```python
from build123d import *

# Parameters (mm, degrees)
SKETCH1_W           = 12
SKETCH1_H           = 10
BOSS_EXTRUDE1_DEPTH = 14.6
SKETCH2_W           = 1
SKETCH2_H           = 5.5
BOSS_EXTRUDE2_DEPTH = 0.5
SKETCH4_R           = 1.5
BOSS_EXTRUDE3_DEPTH = 5.5
SKETCH5_R           = 2.05
BOSS_EXTRUDE4_DEPTH = 0.5
CUT_EXTRUDE1_DEPTH  = 0.5
SKETCH7_R           = 2.5
CUT_EXTRUDE2_DEPTH  = 11
SKETCH9_R           = 3
SKETCH9_R_2         = 2.5
BOSS_EXTRUDE5_DEPTH = 1.6


with BuildPart() as part:
    # Sketch1 → Boss-Extrude1 (new body)
    with BuildSketch(Plane.XY):
        Rectangle(SKETCH1_W, SKETCH1_H)
    extrude(amount=BOSS_EXTRUDE1_DEPTH)

    # Sketch2 → Boss-Extrude2 (add)
    with BuildSketch(Plane.XY.offset(14.6)):
        with Locations((-5.5, 0)):
            Rectangle(SKETCH2_W, SKETCH2_H)
        with Locations((5.5, 0)):
            Rectangle(SKETCH2_W, SKETCH2_H)
    extrude(amount=BOSS_EXTRUDE2_DEPTH)

    # Sketch4 → Boss-Extrude3 (add)
    with BuildSketch(Plane(origin=(0, 0, 0), x_dir=(-1, 0, 0), z_dir=(0, 0, -1))):
        Circle(SKETCH4_R)
    extrude(amount=BOSS_EXTRUDE3_DEPTH)

    # Sketch5 → Boss-Extrude4 (add)
    with BuildSketch(Plane(origin=(0, 0, 0), x_dir=(-1, 0, 0), z_dir=(0, 0, -1))):
        Circle(SKETCH5_R)
    extrude(amount=BOSS_EXTRUDE4_DEPTH)

    # Sketch6 → Cut-Extrude1 (cut)
    with BuildSketch(Plane(origin=(0, 0, 0), x_dir=(-1, 0, 0), z_dir=(0, 0, -1))):
        with BuildLine():
            Line((-5.022000054, 4.19344844), (-4.356935952, 4.19344844))
            Line((-4.356935952, 4.19344844), (-3.752769285, 2.614121517))
            Line((-3.752769285, 2.614121517), (-3.198682747, 4.19344844))
            Line((-3.198682747, 4.19344844), (-2.534820567, 4.19344844))
            Line((-2.534820567, 4.19344844), (-2.534820567, 4.090884337))
            Line((-2.534820567, 4.090884337), (-2.697080183, 4.090884337))
            add(Edge.make_bspline(
                [(-2.697080183, 4.090884337), (-2.710316809, 4.090636556), (-2.734492679, 4.090183998), (-2.76728752, 4.085652982), (-2.793244282, 4.077989549), (-2.813274161, 4.066597021), (-2.826894921, 4.049870677), (-2.8359508, 4.029264042), (-2.841554988, 4.004099098), (-2.842176045, 3.985816116), (-2.842512875, 3.975900363)],
                knots=[0, 0, 0, 0, 1.461409083, 2.669172297, 3.644102285, 4.438396511, 5.171145089, 5.982913306, 6.9060355, 8, 8, 8, 8], degree=3))
            Line((-2.842512875, 3.975900363), (-2.842512875, 2.394570235))
            add(Edge.make_bspline(
                [(-2.842512875, 2.394570235), (-2.842050819, 2.387038144), (-2.841173668, 2.372739479), (-2.834447891, 2.352433769), (-2.823099881, 2.334952111), (-2.806557353, 2.320282642), (-2.784561689, 2.309069969), (-2.756555778, 2.301303429), (-2.722335078, 2.296750977), (-2.697362885, 2.296271709), (-2.683859029, 2.296012542)],
                knots=[0, 0, 0, 0, 0.852734016, 1.618801414, 2.395714484, 3.189123744, 4.096684287, 5.169862416, 6.469586829, 8, 8, 8, 8], degree=3))
            Line((-2.683859029, 2.296012542), (-2.534820567, 2.296012542))
            Line((-2.534820567, 2.296012542), (-2.534820567, 2.19344844))
            Line((-2.534820567, 2.19344844), (-3.432256465, 2.19344844))
            Line((-3.432256465, 2.19344844), (-3.432256465, 2.296012542))
            Line((-3.432256465, 2.296012542), (-3.265189157, 2.296012542))
            add(Edge.make_bspline(
                [(-3.265189157, 2.296012542), (-3.253950106, 2.296245463), (-3.232932895, 2.296681029), (-3.203686174, 2.301738527), (-3.179094381, 2.310536297), (-3.158974617, 2.322618715), (-3.143443119, 2.337663858), (-3.132382481, 2.354803918), (-3.125466503, 2.374031717), (-3.124871883, 2.387565999), (-3.124564157, 2.394570235)],
                knots=[0, 0, 0, 0, 1.394235928, 2.607244209, 3.666761408, 4.619311681, 5.498637875, 6.326439516, 7.133902247, 8, 8, 8, 8], degree=3))
            Line((-3.124564157, 2.394570235), (-3.124564157, 4.09208626))
            Line((-3.124564157, 4.09208626), (-3.791230824, 2.19344844))
            Line((-3.791230824, 2.19344844), (-3.888987234, 2.19344844))
            Line((-3.888987234, 2.19344844), (-4.611743644, 4.08407344))
            Line((-4.611743644, 4.08407344), (-4.611743644, 2.631349081))
            add(Edge.make_bspline(
                [(-4.611743644, 2.631349081), (-4.611377469, 2.611036444), (-4.610694083, 2.573127352), (-4.605325483, 2.520247499), (-4.596108802, 2.475353065), (-4.582524113, 2.437834201), (-4.564432022, 2.407070341), (-4.544422056, 2.379994045), (-4.520414227, 2.357133819), (-4.492696269, 2.33684315), (-4.45794728, 2.320895889), (-4.41471004, 2.309573563), (-4.362603697, 2.300270875), (-4.324529352, 2.297501845), (-4.304051336, 2.296012542)],
                knots=[0, 0, 0, 0, 1.387005521, 2.588542367, 3.624266538, 4.510231893, 5.298685798, 6.05383917, 6.802021236, 7.553697037, 8.390065714, 9.394768359, 10.598794723, 12, 12, 12, 12], degree=3))
            Line((-4.304051336, 2.296012542), (-4.304051336, 2.19344844))
            Line((-4.304051336, 2.19344844), (-5.022000054, 2.19344844))
            Line((-5.022000054, 2.19344844), (-5.022000054, 2.296012542))
            add(Edge.make_bspline(
                [(-5.022000054, 2.296012542), (-5.007558595, 2.297187721), (-4.97993619, 2.299435504), (-4.940384187, 2.30521534), (-4.904363952, 2.311965762), (-4.872178394, 2.321630139), (-4.843002284, 2.331333401), (-4.818185115, 2.344714342), (-4.796055659, 2.35825151), (-4.778051671, 2.375035374), (-4.762204772, 2.393739353), (-4.7498382, 2.416205607), (-4.738151387, 2.44116405), (-4.729866044, 2.469901954), (-4.722344359, 2.501519512), (-4.718026847, 2.536578835), (-4.714468033, 2.57465227), (-4.714362538, 2.601157074), (-4.714307747, 2.614922799)],
                knots=[0, 0, 0, 0, 1.3499974, 2.582161247, 3.724551801, 4.760625632, 5.713431081, 6.581852865, 7.382807722, 8.122943763, 8.865587329, 9.657594863, 10.504338807, 11.429508857, 12.438001628, 13.531119739, 14.71774469, 16, 16, 16, 16], degree=3))
            Line((-4.714307747, 2.614922799), (-4.714307747, 3.992326645))
            add(Edge.make_bspline(
                [(-4.714307747, 3.992326645), (-4.714667267, 4.000376864), (-4.71534259, 4.015498393), (-4.720947722, 4.036459034), (-4.730366107, 4.054081799), (-4.74431361, 4.06851761), (-4.763922895, 4.079141723), (-4.789389281, 4.085827056), (-4.821001443, 4.090114928), (-4.844231256, 4.090612312), (-4.856935952, 4.090884337)],
                knots=[0, 0, 0, 0, 0.964066467, 1.810902258, 2.577654402, 3.336338785, 4.182417323, 5.216170427, 6.47748631, 8, 8, 8, 8], degree=3))
            Line((-4.856935952, 4.090884337), (-5.022000054, 4.090884337))
            Line((-5.022000054, 4.090884337), (-5.022000054, 4.19344844))
        make_face()
    extrude(amount=-CUT_EXTRUDE1_DEPTH, mode=Mode.SUBTRACT)

    # Sketch7 → Cut-Extrude2 (cut)
    with BuildSketch(Plane.XY.offset(14.6)):
        Circle(SKETCH7_R)
    extrude(amount=-CUT_EXTRUDE2_DEPTH, mode=Mode.SUBTRACT)

    # Sketch9 → Boss-Extrude5 (add)
    with BuildSketch(Plane.XY.offset(14.6)):
        with Locations(Location((0, 0, 0), (0, 0, 180))):
            Circle(SKETCH9_R)
        Circle(SKETCH9_R_2, mode=Mode.SUBTRACT)
    extrude(amount=BOSS_EXTRUDE5_DEPTH)

    # Sketch10 → Revolve1 (revolve)
    with BuildSketch(Plane(origin=(0, 0, 0), x_dir=(1, 0, 0), z_dir=(0, 1, 0)), mode=Mode.PRIVATE) as revolve1_sk:
        with BuildLine():
            Line((3.75, -14.6), (3, -14.6))
            Line((3, -14.6), (3, -15.35))
            ThreePointArc((3, -15.35), (3.530330086, -15.130330086), (3.75, -14.6))
        make_face()
    revolve(revolve1_sk.sketch.rotate(Axis((0, 0, 3.6), (0, 0, 1)), 180), axis=Axis((0, 0, 3.6), (0, 0, 1)))


solid = part.part
```
Geometry: final body of the model. Coordinates: model frame, mm. A direction names the side the tool comes from. Coordinates: 2 decimals unless noted, no trailing zeros. Order: outer loops, then holes, each group sorted by start corner. A loop starts at its lowest first (then second) coordinate and runs counter-clockwise, first axis right, second up.
Item 1: Section query D-D (y = -4.25). Output: boundary loops of the cut face in (x, z), then the cut area to 3 significant figures.
Answer:
outline: (-6, 0) - (6, 0) - (6, 14.6) - (-6, 14.6) - close
area: 175 mm2
Item 2: Section query A-A (x = 0). Output: boundary loops of the cut face in (y, z).
Answer:
outline: (-5, 0) - (-2.05, 0) - (-2.05, -0.5) - (-1.5, -0.5) - (-1.5, -5.5) - (1.5, -5.5) - (1.5, -0.5) - (2.05, -0.5) - (2.05, 0) - (5, 0) - (5, 14.6) - (3.75, 14.6) arc R0.75 ccw to (3, 15.35) - (3, 16.2) - (2.5, 16.2) - (2.5, 3.6) - (-2.5, 3.6) - (-2.5, 16.2) - (-3, 16.2) - (-3, 15.35) arc R0.75 ccw to (-3.75, 14.6) - (-5, 14.6) - close
Item 3: Section query C-C (z = -1.5). Output: boundary loops of the cut face in (x, y), then the cut area to 3 significant figures.
Answer:
outline: circle Ø3 at (0, 0)
area: 7.07 mm2
Item 4: Material intervals for line 1 along Y through (x, z) = (0, 6.5); line 2 along Z through (x, y) = (2.75, 0.5); line 3 along Z through (x, y) = (4.5, 0.5), sorted ascending.
Answer:
line 1: y = -5 to -2.5, 2.5 to 5
line 2: z = 0 to 16.2
line 3: z = 0 to 14.6
Item 5: Draft query along X for faces 6 (the face through (0, 0, 3.6)), 7 (the face through (1.5, 0.07, -2.96)), 8 (the face through (-0.54, -2.44, 9.81)), 9 (the face through (2, -2, 16.2)). Return one class per face: released by +X, released by -X, zero draft, split by the parting line, or undercut.
Answer:
face 6: undercut
face 7: split by the parting line
face 8: undercut
face 9: zero draft
Item 6: Section query B-B (y = 0). Output: boundary loops of the cut face in (x, z), then the cut area to 3 significant figures.
Answer:
outline: (-6, 0) - (-2.05, 0) - (-2.05, -0.5) - (-1.5, -0.5) - (-1.5, -5.5) - (1.5, -5.5) - (1.5, -0.5) - (2.05, -0.5) - (2.05, 0) - (6, 0) - (6, 15.1) - (5, 15.1) - (5, 14.6) - (3.75, 14.6) arc R0.75 ccw to (3, 15.35) - (3, 16.2) - (2.5, 16.2) - (2.5, 3.6) - (-2.5, 3.6) - (-2.5, 16.2) - (-3, 16.2) - (-3, 15.35) arc R0.75 ccw to (-3.75, 14.6) - (-5, 14.6) - (-5, 15.1) - (-6, 15.1) - close
area: 141 mm2
Item 7: Contact query for flat-ended pins moving along their axis: P1, Ø0.6, axis at x = 4, y = 3.5, coming from the -Z side; P2, Ø4.5, axis at x = 0, y = 0, coming from the +Z side. Output: stop coordinate, or through.
Answer:
P1: stops at z = 0
P2: stops at z = 3.6
Item 8: Access query for faces 1 (the face through (-2.86, -0.9, 15.77)), 2 (the face through (-0.1, -2.2, 0)), 3 (the face through (0, 0, -5.5)), 4 (the face through (-5.5, 0, 15.1)), 5 (the face through (5.5, 0, 15.1)). Directions: +Z, -Z, +X, -X, +Y, -Y. A direction counts if a zero-diameter tool reaches every point of the face in a straight line with its end or side. Return the directions, or none.
Answer:
face 1: +Z
face 2: -Z
face 3: -Z, +X, -X, +Y, -Y
face 4: +Z, -X, +Y, -Y
face 5: +Z, +X, +Y, -Y
